Build history of the part. All positions in model axes, mm. Face numbers are marked on the shaded views. A direction names the side the tool comes from. Give positions to 0.01 mm unless a question says otherwise; leave off trailing zeros. Order: outer loops, then holes, each group sorted by start corner. A loop starts at its lowest first (then second) coordinate and runs counter-clockwise, first axis right, second up. Notation, with made-up numbers: (-34, 48.5) - (-7, 48.5) arc R24 cw to (-7, 59.5) - close; hole circle Ø9 at (70.25, 60). An arc over 180 degrees is marked (long way). One line per item, written item: value.
Autodesk Inventor part; units mm, degrees
ref_plane "Work Plane1" through (0, 500, 0) normal (0, 1, 0) x (1, 0, 0)
ref_plane "YZ Plane" through (0, 0, 0) normal (1, 0, 0) x (0, 1, 0)
ref_plane "XZ Plane" through (0, 0, 0) normal (0, 1, 0) x (-1, 0, 0)
sketch "Sketch1" plane through (0, 0, 0) normal (0, 1, 0) x (-1, 0, 0)
  circle A0 centre (-83.0821, 235.7909) radius 5
  circle A1 centre (-162.6599, -189.8467) radius 5
  circle A2 centre (245.742, -45.9443) radius 5
  point P0 (0, 0)
  dimension "d3" = 10
  dimension "d4" = 10
  dimension "d5" = 10
extrude "Extrusion1" add sketch "Sketch1" along normal blind 750
sketch "Sketch2" plane through (83.0821, 750, 235.7909) normal (0, 1, 0) x (1, 0, 0)
  circle A0 centre (-328.8241, 281.7352) radius 5
  circle A1 centre (79.5778, 425.6376) radius 5
  line L0 (-326.9753, 276.3685) -> (-84.2277, 230.0921)
  line L1 (-82.7079, 228.7691) -> (-5.5677, 1.0437)
  circle A2 centre (0, 0) radius 5
  line L2 (-325.1511, 286.0493) -> (-86.7137, 240.5946)
  line L3 (-86.7137, 240.5946) -> (74.0056, 426.7207)
  line L4 (81.481, 420.2957) -> (-74.7837, 239.3284)
  line L5 (-75.1642, 237.3796) -> (3.7927, 4.2915)
  arc A3 (-327.4871, 284.4754) -> (-328.5709, 278.6773) centre (-83.0821, 235.7909) ccw
  arc A4 (-3.0309, -0.2086) -> (2.5859, 1.7717) centre (-83.0821, 235.7909) ccw
  arc A5 (81.2864, 423.1061) -> (76.8025, 426.9477) centre (-83.0821, 235.7909) ccw
  arc A6 (-82.7079, 228.7691) -> (-84.2277, 230.0921) centre (-84.6022, 228.1275) ccw
  arc A7 (76.8025, 426.9477) -> (74.0056, 426.7207) centre (75.5193, 425.4136) ccw
  arc A8 (81.481, 420.2957) -> (81.2864, 423.1061) centre (79.9673, 421.6028) ccw
  arc A9 (2.5859, 1.7717) -> (3.7927, 4.2915) centre (1.8984, 3.6499) ccw
  arc A10 (-5.5677, 1.0437) -> (-3.0309, -0.2086) centre (-3.6734, 1.6854) ccw
  arc A11 (-74.7837, 239.3284) -> (-75.1642, 237.3796) centre (-73.2699, 238.0212) ccw
  arc A12 (-328.5709, 278.6773) -> (-326.9753, 276.3685) centre (-326.6007, 278.3331) ccw
  arc A13 (-325.1511, 286.0493) -> (-327.4871, 284.4754) centre (-325.5257, 284.0846) ccw
  point P0 (-83.0821, 235.7909)
  point P1 (-328.9022, 276.7358)
  point P2 (-4.9283, -0.8437)
  point P3 (75.2872, 428.2049)
  point P4 (82.7726, 421.7915)
  point P5 (-75.5311, 238.4628)
  point P6 (4.4165, 2.45)
  dimension "d8" = 2
  dimension "d9" = 2
extrude "Extrusion2" add sketch "Sketch2" against normal blind 10 contours A0 A12 A3 A13 | A0 A13 L2 L3 A7 A1 A8 L4 A11 L5 A9 A2 A10 L1 A6 L0 A12 | A7 A5 A8 A1 | A2 A9 A4 A10 picked at (-326.6818, 281.2494) picked at (78.1424, 423.9745) picked at (-0.6818, 2.0889)
ref_plane "Work Plane1" through (0, 500, 0) normal (0, 1, 0) x (1, 0, 0)
mirror "Mirror1" about plane through (0, 500, 0) normal (0, 1, 0) of "Extrusion2"
sketch "Sketch3" plane through (0, 750, 0) normal (0, 1, 0) x (1, 0, 0)
  circle A0 centre (0, 0) radius 125
  dimension "d13" = 250
extrude "Extrusion3" add sketch "Sketch3" along normal blind 1
mirror "Mirror2" about plane through (0, 500, 0) normal (0, 1, 0) of "Extrusion3"
sketch "Sketch4" plane through (0, 500, 0) normal (0, 1, 0) x (1, 0, 0)
  circle A0 centre (0, 0) radius 252.3793
  circle A1 centre (0, 0) radius 125
extrude "Extrusion5" add sketch "Sketch4" along normal blind 1 contours A0 | A1
sketch "Sketch5" plane through (0, 501, 0) normal (0, 1, 0) x (1, 0, 0)
  circle A0 centre (3.3929, 3.4645) radius 124.3815
  point P0 (0, 0)
extrude "Extrusion6" cut sketch "Sketch5" against normal blind 1
properties part number "boiler_plates"
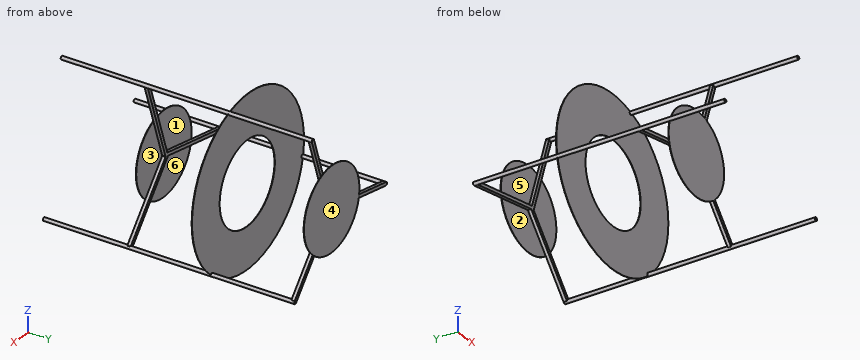
(1) Drill centre lines: line 1 (Y direction, x = -46, z = -63); line 2 (Y direction, x = 21, z = 216); line 3 (Z direction, x = 84.5, y = 137.5). Where is each one in solid material? Low to high.
Completed:
line 1: 249 to 250, 750 to 751
line 2: 500 to 501
line 3: 231 to 240.59
(2) Slice it at D-D, the plane y = 635.5. Give the cut face in (x, z), and give its area (3 significant figures).
Completed:
outline: circle Ø10 at (-245.74, -45.94); circle Ø10 at (83.08, 235.79); circle Ø10 at (162.66, -189.85)
area: 236 mm²
(3) Pin check, flat tips, straight feed: P1, Ø1.5, axis at x = 99.5, z = 155, coming from the +Y side; P2, Ø8, axis at x = 78.5, y = 567, coming from the +Z side; P3, Ø1, axis at x = 5.5, z = -66.5, coming from the -Y side. Stop position of each tip, or through.
Completed:
P1: y = 501
P2: z = 240.76
P3: y = 249
(4) Slice it at C-C, the plane x = -112. Give the cut face in (y, z).
Completed:
outline: (249, -55.51) - (250, -55.51) - (250, -25.46) - (260, -25.46) - (260, -15.43) - (250, -15.43) - (250, 55.51) - (249, 55.51) - close; (500, -226.17) - (501, -226.17) - (501, -49.89) - (500, -49.89) - close; (500, 42.96) - (501, 42.96) - (501, 226.17) - (500, 226.17) - close; (740, -25.46) - (750, -25.46) - (750, -55.51) - (751, -55.51) - (751, 55.51) - (750, 55.51) - (750, -15.43) - (740, -15.43) - close
(5) Slice it at B-B, the plane z = -147. Give the cut face in (x, y).
Completed:
outline: (-205.15, 500) - (205.15, 500) - (205.15, 501) - (-205.15, 501) - close; (119.15, 250) - (132.18, 250) - (132.18, 260) - (119.15, 260) - close; (119.15, 740) - (132.18, 740) - (132.18, 750) - (119.15, 750) - close
(6) 3-axis set-ups, long thin cutter, end or side, ignore diameter. For the marked faces 1, 2, 3 and 4: which of +Z, -Z, +X, -X, +Y, -Y reach the whole face in a straight line?
Completed:
face 1: +Z, -X
face 2: -Z
face 3: +X
face 4: +Z, -Z, +X, -X, +Y
(7) Pull direction X, two halves, no side cores. Call the marked faces 5 and 6: +X half, -X half, draft (parallel to the pull), parting line (faces both ways), or undercut.
Completed:
face 5: draft
face 6: undercut
(8) Slice it at A-A, the plane x = -163.5. Give the cut face in (y, z).
Completed:
outline: (250, -35.28) - (260, -35.28) - (260, -25.25) - (250, -25.25) - close; (500, -192.26) - (501, -192.26) - (501, 192.26) - (500, 192.26) - close; (740, -35.28) - (750, -35.28) - (750, -25.25) - (740, -25.25) - close
